```python
from build123d import *

# Parameters (mm, degrees)
SKETCH1_W           = 45
SKETCH1_H           = 50
BOSS_EXTRUDE1_DEPTH = 45
SKETCH2_R           = 5.2
CUT_EXTRUDE1_DEPTH  = 45
SKETCH9_R           = 5.15
CUT_EXTRUDE6_DEPTH  = 2
SKETCH10_R          = 5.15
CUT_EXTRUDE7_DEPTH  = 2
SKETCH12_R          = 12.7
CUT_EXTRUDE8_DEPTH  = 46
SKETCH13_W          = 45
SKETCH13_H          = 6.66747138
CUT_EXTRUDE9_DEPTH  = 46
SKETCH16_R          = 13.25
SKETCH16_R_2        = 3.75
BOSS_EXTRUDE3_DEPTH = 2
FILLET1_R           = 10
SKETCH17_R          = 1.6
CUT_EXTRUDE10_DEPTH = 10
SKETCH18_R          = 2.4
CUT_EXTRUDE11_DEPTH = 1


with BuildPart() as part:
    # Sketch1 → Boss-Extrude1 (new body)
    with BuildSketch(Plane.XY):
        with Locations((8.236607143, -2.901785714)):
            Rectangle(SKETCH1_W, SKETCH1_H)
    extrude(amount=BOSS_EXTRUDE1_DEPTH)

    # Sketch2 → Cut-Extrude1 (cut)
    with BuildSketch(Plane.XY.offset(45)):
        with Locations((-4.163392857, -24.901785714)):
            Circle(SKETCH2_R)
        with Locations((20.636607143, -24.901785714)):
            Circle(SKETCH2_R)
    extrude(amount=-CUT_EXTRUDE1_DEPTH, mode=Mode.SUBTRACT)

    # Sketch9 → Cut-Extrude6 (cut)
    with BuildSketch(Plane.XY.offset(45)):
        with Locations((8.236607143, -2.401785714)):
            Circle(SKETCH9_R)
    extrude(amount=-CUT_EXTRUDE6_DEPTH, mode=Mode.SUBTRACT)

    # Sketch10 → Cut-Extrude7 (cut)
    with BuildSketch(Plane(origin=(0, 0, 0), x_dir=(-1, 0, 0), z_dir=(0, 0, -1))):
        with Locations((-8.236607143, -2.401785714)):
            Circle(SKETCH10_R)
    extrude(amount=-CUT_EXTRUDE7_DEPTH, mode=Mode.SUBTRACT)

    # Sketch12 → Cut-Extrude8 (cut)
    with BuildSketch(Plane.ZY.offset(14.263392857)):
        with Locations((22.5, 0)):
            Circle(SKETCH12_R)
    extrude(amount=-CUT_EXTRUDE8_DEPTH, mode=Mode.SUBTRACT)

    # Sketch13 → Cut-Extrude9 (cut)
    with BuildSketch(Plane.ZY.offset(14.263392857)):
        with Locations((22.5, 18.764478596)):
            Rectangle(SKETCH13_W, SKETCH13_H)
    extrude(amount=-CUT_EXTRUDE9_DEPTH, mode=Mode.SUBTRACT)

    # Sketch16 → Boss-Extrude3 (add)
    with BuildSketch(Plane(origin=(30.736607143, 0, 0), x_dir=(0, 0, -1), z_dir=(1, 0, 0))):
        with Locations((-22.5, 0)):
            Circle(SKETCH16_R)
        with Locations((-22.5, 0)):
            Circle(SKETCH16_R_2, mode=Mode.SUBTRACT)
    extrude(amount=-BOSS_EXTRUDE3_DEPTH)

    # Fillet1
    fillet1_edges = [part.edges().sort_by_distance(p)[0] for p in [
        (8.236607143, 15.430742906, 0),
        (8.236607143, 15.430742906, 45),
    ]]
    fillet(fillet1_edges, radius=FILLET1_R)

    # Sketch17 → Cut-Extrude10 (cut)
    with BuildSketch(Plane(origin=(30.736607143, 0, 0), x_dir=(0, 0, -1), z_dir=(1, 0, 0))):
        with Locations((-22.5, 8)):
            Circle(SKETCH17_R)
    extrude(amount=-CUT_EXTRUDE10_DEPTH, mode=Mode.SUBTRACT)

    # Sketch18 → Cut-Extrude11 (cut)
    with BuildSketch(Plane(origin=(30.736607143, 0, 0), x_dir=(0, 0, -1), z_dir=(1, 0, 0))):
        with Locations((-22.5, 8)):
            Circle(SKETCH18_R)
    extrude(amount=-CUT_EXTRUDE11_DEPTH, mode=Mode.SUBTRACT)


solid = part.part
```
The model under review builds one solid part; all positions refer to its coordinate system, in mm. A direction names the side the tool comes from. Coordinates: 2 decimals unless noted, no trailing zeros. Write each loop counter-clockwise with the first axis right and the second up, starting at its lowest first coordinate (ties: lowest second). Pieces come first, ordered by that corner, then holes. Notation, with made-up numbers: (-11, 62.5) -> (14, 62.5) arc R23 ccw to (14, 91.5) -> close; hole circle Ø2 at (10, 45.5). An arc over 180 degrees is marked (long way). One line per item, written item: value. Start each with the question number.
Q1. Clearance check with flat-ended pins moving along their axes: P1, Ø3, axis at x = 10.5, y = -3.5, coming from the -Z side; P2, Ø10, axis at x = 7, y = 7, coming from the +Z side; P3, Ø8, axis at x = 8.24, y = -2.4, coming from the +Z side; P4, Ø4, axis at y = 8, z = 22.5, coming from the +X side. State where each tip first meets the part, or that it passes through.
Q2. The part is to be moulded in two halves that separate along Z. For faces 6 (the face through (30.737, -7, 22)), 7 (the face through (6.936, 3.815, 34.614)), 8 (the face through (8, -11, 0)), say which applies: +Z half, -Z half, draft (parallel to the pull), parting line (faces both ways), or undercut.
Q3. Add section A-A, the plane z = 22.5. Give the boundary of the cut face in (x, y).
Q4. To check wall thickness, follow probe 1 along Y at (x, z) = (30.05, 22.5); probe 2 along Y at (x, z) = (29.3, 22.5); probe 3 along X at (y, z) = (-25, 3.5). State the ranges of each line that lie inside material, in increasing order.
Q5. For faces 1 (the face through (3.324, -0.855, 0.986)), 2 (the face through (8.55, 12.58, 41.99)), 3 (the face through (29.737, 6, 22)), 4 (the face through (4.44, 1.08, 44.01)), 5 (the face through (8.55, 12.42, 2.85)), list the 3-axis set-ups (+Z, -Z, +X, -X, +Y, -Y) from which the entire face can be reached by the end or side of a thin tool; tool diameter is ignored.
Q6. Add section B-B, the plane y = 8. Give the boundary of the cut face in (x, z).
Q7. Add section C-C, the plane y = -23.5. Give the boundary of the cut face in (x, z), then the cut area to 3 significant figures.
Q8. Add section D-D, the plane x = 8. Give the boundary of the cut face in (y, z).
Response:
1. P1: z = 2
1. P2: z = 45
1. P3: z = 43
1. P4: x = 29.74
2. face 6: draft
2. face 7: undercut
2. face 8: -Z half
3. outline: (-14.26, -27.9) -> (-8.41, -27.9) arc R5.2 cw (long way) to (0.08, -27.9) -> (16.39, -27.9) arc R5.2 cw (long way) to (24.88, -27.9) -> (30.74, -27.9) -> (30.74, -3.75) -> (28.74, -3.75) -> (28.74, -12.7) -> (-14.26, -12.7) -> close; (-14.26, 12.7) -> (28.74, 12.7) -> (28.74, 9.6) -> (29.74, 9.6) -> (29.74, 10.4) -> (30.74, 10.4) -> (30.74, 15.43) -> (-14.26, 15.43) -> close; (28.74, 3.75) -> (30.74, 3.75) -> (30.74, 5.6) -> (29.74, 5.6) -> (29.74, 6.4) -> (28.74, 6.4) -> close
4. probe 1: -27.9 to -3.75, 3.75 to 5.6, 10.4 to 15.43
4. probe 2: -27.9 to -3.75, 3.75 to 6.4, 9.6 to 15.43
4. probe 3: -14.26 to -9.36, 1.04 to 15.44, 25.84 to 30.74
5. face 1: -Z
5. face 2: +Z, +X, -X, +Y
5. face 3: +X
5. face 4: +Z
5. face 5: -Z, +X, -X, +Y
6. outline: (-14.26, 0.34) -> (30.74, 0.34) -> (30.74, 20.1) -> (29.74, 20.1) -> (29.74, 20.9) -> (28.74, 20.9) -> (28.74, 12.64) -> (-14.26, 12.64) -> close; (-14.26, 32.36) -> (28.74, 32.36) -> (28.74, 24.1) -> (29.74, 24.1) -> (29.74, 24.9) -> (30.74, 24.9) -> (30.74, 44.66) -> (-14.26, 44.66) -> close
7. outline: (-14.26, 0) -> (-9.17, 0) -> (-9.17, 45) -> (-14.26, 45) -> close; (0.84, 0) -> (15.63, 0) -> (15.63, 45) -> (0.84, 45) -> close; (25.64, 0) -> (30.74, 0) -> (30.74, 45) -> (25.64, 45) -> close
7. area: 1,120 mm²
8. outline: (-27.9, 0) -> (-7.55, 0) -> (-7.55, 2) -> (2.74, 2) -> (2.74, 0) -> (5.43, 0) arc R10 ccw to (15.43, 10) -> (15.43, 35) arc R10 ccw to (5.43, 45) -> (2.74, 45) -> (2.74, 43) -> (-7.55, 43) -> (-7.55, 45) -> (-27.9, 45) -> close; hole circle Ø25.4 at (0, 22.5)
